Could you check a few things on this model? Use its own coordinates, in mm. A direction names the side the tool comes from. Coordinates: 2 decimals unless noted, no trailing zeros. Loops run counter-clockwise (first coordinate to the right, second up) from the corner with the lowest first, then second, coordinate; pieces in that order, holes last. Notation, with made-up numbers: (67, -27.5) - (76, -27.5) arc R32 cw to (76, -0.5) - close; hole circle Ø10 at (17.5, -26.75). An arc over 180 degrees is marked (long way). One line per question, with ' | ' between items. Start each with the question number.
1. I want a section at C-C, the plane z = 5. Write out the boundary of the cut face in (x, y), then the cut area to 3 significant figures.
2. I want a section at A-A, the plane z = 0. Write out the boundary of the cut face in (x, y), then the cut area to 3 significant figures.
3. Which directions (+Z, -Z, +X, -X, +Y, -Y) give clear straight access to the entire face, cutting with the end or side of a thin tool? Please do faces 1 (the cylindrical face through (5.41, -38.49, -3.86)), 2 (the flat face through (0, -18, -9.65)).
4. I want a section at D-D, the plane x = -15. Write out the boundary of the cut face in (y, z).
5. Please list where these lines run through material, in increasing order: L1, parallel to Y at x = -11.5, z = -7.75; L2, parallel to Y at x = 12.5, z = 3.75; L3, parallel to Z at x = 11, y = -38. Write a range as [from, to].
6. I'm going to push flat-ended pins straight in: P1, Ø1, axis at x = 6, z = 1, coming from the -Y side; P2, Ø3, axis at x = -2, z = -4, coming from the -Y side. Where does each tip first touch, or does it pass through?
7. I want a section at B-B, the plane x = 10.45. Write out the boundary of the cut face in (y, z), then the cut area to 3 significant figures.
from build123d import *

# Parameters (mm, degrees)
F0_W     = 40.6
F0_H     = 19.3
F1_DEPTH = 37.5
F2_R     = 6.35
F3_DEPTH = 2
F4_R     = 2.85
F5_DEPTH = 4


with BuildPart() as f1:
    # F0 (on Front) → F1 (new body)
    with BuildSketch(Plane.XZ):
        Rectangle(F0_W, F0_H)
    extrude(amount=F1_DEPTH)

    # F2 (on face) → F3 (join)
    with BuildSketch(Plane.XZ.offset(37.5)):
        with Locations((10.45, 0)):
            Circle(F2_R)
    extrude(amount=F3_DEPTH)

    # F4 (on face) → F5 (join)
    with BuildSketch(Plane.XZ.offset(39.5)):
        with Locations((10.45, 0)):
            Circle(F4_R)
    extrude(amount=F5_DEPTH)


solid = f1.part
Results are:
1) outline: (-20.3, -37.5) - (6.54, -37.5) - (6.54, -39.5) - (14.36, -39.5) - (14.36, -37.5) - (20.3, -37.5) - (20.3, 0) - (-20.3, 0) - close | area: 1,540 mm2
2) outline: (-20.3, -37.5) - (4.1, -37.5) - (4.1, -39.5) - (7.6, -39.5) - (7.6, -43.5) - (13.3, -43.5) - (13.3, -39.5) - (16.8, -39.5) - (16.8, -37.5) - (20.3, -37.5) - (20.3, 0) - (-20.3, 0) - close | area: 1,570 mm2
3) face 1: -Y | face 2: -Z, +X, -X, +Y, -Y
4) outline: (-37.5, -9.65) - (0, -9.65) - (0, 9.65) - (-37.5, 9.65) - close
5) L1: y = [-37.5, 0] | L2: y = [-39.5, 0] | L3: z = [-6.33, 6.33]
6) P1: stops at y = -39.5 | P2: stops at y = -37.5
7) outline: (-43.5, -2.85) - (-39.5, -2.85) - (-39.5, -6.35) - (-37.5, -6.35) - (-37.5, -9.65) - (0, -9.65) - (0, 9.65) - (-37.5, 9.65) - (-37.5, 6.35) - (-39.5, 6.35) - (-39.5, 2.85) - (-43.5, 2.85) - close | area: 772 mm2
